```python
from build123d import *

# Parameters (mm, degrees)
SKETCH_1_W             = 23.5
SKETCH_1_H             = 12
EXTRUDE_1_DEPTH        = 771
HOLE_WIZARD_M6_1_D     = 5
HOLE_WIZARD_M6_1_DEPTH = 15
HOLE_WIZARD_M6_1_TIP   = 1.502151548
HOLE_WIZARD_M6_2_D     = 5
HOLE_WIZARD_M6_2_DEPTH = 15
HOLE_WIZARD_M6_2_TIP   = 1.502151548
SKETCH_7_R             = 4.5
CUT_EXTRUDE_1_DEPTH    = 772.729227126
SKETCH_8_R             = 5
CUT_EXTRUDE_2_DEPTH    = 15
SKETCH_9_R             = 3.5
CUT_EXTRUDE_3_DEPTH    = 15
HOLE_WIZARD_M6_3_D     = 5
HOLE_WIZARD_M6_3_DEPTH = 15
HOLE_WIZARD_M6_3_TIP   = 1.502151548
HOLE_WIZARD_M6_4_D     = 5
HOLE_WIZARD_M6_4_DEPTH = 15
HOLE_WIZARD_M6_4_TIP   = 1.502151548
SKETCH_14_R            = 4.5
CUT_EXTRUDE_4_DEPTH    = 772.729227126


with BuildPart() as part:
    # 草图1 → 凸台-拉伸1 (new, symmetric)
    with BuildSketch(Plane(origin=(0, 0, 0), x_dir=(0, 0, -1), z_dir=(1, 0, 0))):
        with BuildLine():
            Line((-14, 15), (-11.5, 15))
            Line((-11.5, 15), (-11.5, 13.5))
            Line((-11.5, 13.5), (-11.4, 13.5))
            ThreePointArc((-11.4, 13.5), (-11.117157288, 13.382842712), (-11, 13.1))
            Line((-11, 13.1), (-11, 12))
            Line((-11, 12), (-9.5, 12))
            Line((-9.5, 12), (-9.5, 15))
            Line((-9.5, 15), (-8, 15))
            Line((-8, 15), (-8, 12.5))
            Line((-8, 12.5), (-5, 12.5))
            Line((-5, 12.5), (-5, 15))
            Line((-5, 15), (5, 15))
            Line((5, 15), (5, 12.5))
            Line((5, 12.5), (8, 12.5))
            Line((8, 12.5), (8, 15))
            Line((8, 15), (9.5, 15))
            Line((9.5, 15), (9.5, 12))
            Line((9.5, 12), (11, 12))
            Line((11, 12), (11, 13.1))
            ThreePointArc((11, 13.1), (11.117157288, 13.382842712), (11.4, 13.5))
            Line((11.4, 13.5), (11.5, 13.5))
            Line((11.5, 13.5), (11.5, 15))
            Line((11.5, 15), (14, 15))
            ThreePointArc((14, 15), (14.707106781, 14.707106781), (15, 14))
            Line((15, 14), (15, 8))
            Line((15, 8), (12.5, 8))
            Line((12.5, 8), (12.5, 5))
            Line((12.5, 5), (15, 5))
            Line((15, 5), (15, -5))
            Line((15, -5), (12.5, -5))
            Line((12.5, -5), (12.5, -8))
            Line((12.5, -8), (15, -8))
            Line((15, -8), (15, -14))
            ThreePointArc((15, -14), (14.707106781, -14.707106781), (14, -15))
            Line((14, -15), (11.5, -15))
            Line((11.5, -15), (11.5, -13.5))
            Line((11.5, -13.5), (11.4, -13.5))
            ThreePointArc((11.4, -13.5), (11.117157288, -13.382842712), (11, -13.1))
            Line((11, -13.1), (11, -12))
            Line((11, -12), (9.5, -12))
            Line((9.5, -12), (9.5, -15))
            Line((9.5, -15), (8, -15))
            Line((8, -15), (8, -12.5))
            Line((8, -12.5), (5, -12.5))
            Line((5, -12.5), (5, -15))
            Line((5, -15), (-5, -15))
            Line((-5, -15), (-5, -12.5))
            Line((-5, -12.5), (-8, -12.5))
            Line((-8, -12.5), (-8, -15))
            Line((-8, -15), (-9.5, -15))
            Line((-9.5, -15), (-9.5, -12))
            Line((-9.5, -12), (-11, -12))
            Line((-11, -12), (-11, -13.1))
            ThreePointArc((-11, -13.1), (-11.117157288, -13.382842712), (-11.4, -13.5))
            Line((-11.4, -13.5), (-11.5, -13.5))
            Line((-11.5, -13.5), (-11.5, -15))
            Line((-11.5, -15), (-14, -15))
            ThreePointArc((-14, -15), (-14.707106781, -14.707106781), (-15, -14))
            Line((-15, -14), (-15, 14))
            ThreePointArc((-15, 14), (-14.707106781, 14.707106781), (-14, 15))
        make_face()
        with BuildLine():
            Line((12, -10.5), (12, -8.5))
            ThreePointArc((12, -8.5), (11.853553391, -8.146446609), (11.5, -8))
            Line((11.5, -8), (-11.5, -8))
            ThreePointArc((-11.5, -8), (-11.853553391, -8.146446609), (-12, -8.5))
            Line((-12, -8.5), (-12, -10.5))
            ThreePointArc((-12, -10.5), (-11.853553391, -10.853553391), (-11.5, -11))
            Line((-11.5, -11), (11.5, -11))
            ThreePointArc((11.5, -11), (11.853553391, -10.853553391), (12, -10.5))
        make_face(mode=Mode.SUBTRACT)
        with BuildLine():
            Line((-11.5, 11), (11.5, 11))
            ThreePointArc((11.5, 11), (11.853553391, 10.853553391), (12, 10.5))
            Line((12, 10.5), (12, 8.5))
            ThreePointArc((12, 8.5), (11.853553391, 8.146446609), (11.5, 8))
            Line((11.5, 8), (-11.5, 8))
            ThreePointArc((-11.5, 8), (-11.853553391, 8.146446609), (-12, 8.5))
            Line((-12, 8.5), (-12, 10.5))
            ThreePointArc((-12, 10.5), (-11.853553391, 10.853553391), (-11.5, 11))
        make_face(mode=Mode.SUBTRACT)
        Rectangle(SKETCH_1_W, SKETCH_1_H, mode=Mode.SUBTRACT)
    extrude(amount=EXTRUDE_1_DEPTH, both=True)

    # M6 螺纹孔1
    with Locations(Plane(origin=(0, 0, -15), x_dir=(-1, 0, 0), z_dir=(0, 0, -1))):
        with Locations((751, 0), (736, 0), (-736, 0), (-751, 0)):
            Hole(HOLE_WIZARD_M6_1_D / 2, depth=HOLE_WIZARD_M6_1_DEPTH)
            with Locations((0, 0, -(HOLE_WIZARD_M6_1_DEPTH + HOLE_WIZARD_M6_1_TIP / 2))):  # 118° drill point
                Cone(0, HOLE_WIZARD_M6_1_D / 2, HOLE_WIZARD_M6_1_TIP, mode=Mode.SUBTRACT)

    # M6 螺纹孔2
    with Locations(Plane(origin=(0, 15, 0), x_dir=(-1, 0, 0), z_dir=(0, 1, 0))):
        with Locations((-751, 0), (-736, 0), (736, 0), (751, 0)):
            Hole(HOLE_WIZARD_M6_2_D / 2, depth=HOLE_WIZARD_M6_2_DEPTH)
            with Locations((0, 0, -(HOLE_WIZARD_M6_2_DEPTH + HOLE_WIZARD_M6_2_TIP / 2))):  # 118° drill point
                Cone(0, HOLE_WIZARD_M6_2_D / 2, HOLE_WIZARD_M6_2_TIP, mode=Mode.SUBTRACT)

    # 草图7 → 切除-拉伸1 (cut, through all)
    with BuildSketch(Plane.XY.offset(15)):
        with Locations((-651, 0)):
            Circle(SKETCH_7_R)
        with Locations((-221, 0)):
            Circle(SKETCH_7_R)
        with Locations((651, 0)):
            Circle(SKETCH_7_R)
        with Locations((221, 0)):
            Circle(SKETCH_7_R)
    extrude(amount=-CUT_EXTRUDE_1_DEPTH, mode=Mode.SUBTRACT)

    # 草图8 → 切除-拉伸2 (cut)
    with BuildSketch(Plane.XY.offset(15)):
        Circle(SKETCH_8_R)
        with Locations((-25, 0)):
            Circle(SKETCH_8_R)
        with Locations((25, 0)):
            Circle(SKETCH_8_R)
    extrude(amount=-CUT_EXTRUDE_2_DEPTH, mode=Mode.SUBTRACT)

    # 草图9 → 切除-拉伸3 (cut)
    with BuildSketch(Plane(origin=(0, 0, -15), x_dir=(-1, 0, 0), z_dir=(0, 0, -1))):
        Circle(SKETCH_9_R)
        with BuildLine():
            Line((27, 2.5), (27, -2.5))
            ThreePointArc((27, -2.5), (25, -4.5), (23, -2.5))
            Line((23, -2.5), (23, 2.5))
            ThreePointArc((23, 2.5), (25, 4.5), (27, 2.5))
        make_face()
        with BuildLine():
            Line((-27, 2.5), (-27, -2.5))
            ThreePointArc((-27, -2.5), (-25, -4.5), (-23, -2.5))
            Line((-23, -2.5), (-23, 2.5))
            ThreePointArc((-23, 2.5), (-25, 4.5), (-27, 2.5))
        make_face()
    extrude(amount=-CUT_EXTRUDE_3_DEPTH, mode=Mode.SUBTRACT)

    # M6 螺纹孔3
    with Locations(Plane(origin=(0, 0, -15), x_dir=(-1, 0, 0), z_dir=(0, 0, -1))):
        with Locations((411, 0), (351, 0), (321, 0), (261, 0), (-261, 0), (-321, 0), (-351, 0), (-411, 0)):
            Hole(HOLE_WIZARD_M6_3_D / 2, depth=HOLE_WIZARD_M6_3_DEPTH)
            with Locations((0, 0, -(HOLE_WIZARD_M6_3_DEPTH + HOLE_WIZARD_M6_3_TIP / 2))):  # 118° drill point
                Cone(0, HOLE_WIZARD_M6_3_D / 2, HOLE_WIZARD_M6_3_TIP, mode=Mode.SUBTRACT)

    # M6 螺纹孔4
    with Locations(Plane(origin=(0, 0, -15), x_dir=(-1, 0, 0), z_dir=(0, 0, -1))):
        with Locations((691, 0), (-691, 0)):
            Hole(HOLE_WIZARD_M6_4_D / 2, depth=HOLE_WIZARD_M6_4_DEPTH)
            with Locations((0, 0, -(HOLE_WIZARD_M6_4_DEPTH + HOLE_WIZARD_M6_4_TIP / 2))):  # 118° drill point
                Cone(0, HOLE_WIZARD_M6_4_D / 2, HOLE_WIZARD_M6_4_TIP, mode=Mode.SUBTRACT)

    # 草图14 → 切除-拉伸4 (cut, through all)
    with BuildSketch(Plane(origin=(0, 0, -15), x_dir=(-1, 0, 0), z_dir=(0, 0, -1))):
        with Locations((691, 0)):
            Circle(SKETCH_14_R)
        with Locations((-691, 0)):
            Circle(SKETCH_14_R)
    extrude(amount=-CUT_EXTRUDE_4_DEPTH, mode=Mode.SUBTRACT)


solid = part.part
```
Check sheet for the modelled part. Datum: model origin and axes. Units: mm. A direction names the side the tool comes from. Give positions to 0.01 mm unless a question says otherwise; leave off trailing zeros. Use CSV: the item, a comma, the result in double quotes. Start each with the question number.
1) Set-up check for faces 3 (the face through (771, 7, 0)), 4 (the face through (11, -6, 0)): record each of +Z, -Z, +X, -X, +Y, -Y from which the full face is reachable in a straight line by a thin tool's end or side.
2) Material ranges on line 1 (Y direction, x = -178.5, z = -4); line 2 (Y direction, x = 201.5, z = -5.5); line 3 (Z direction, x = 39, y = 13.75), recorded low to high. Write a range as from..to.
3) Go/stop test with flat-tipped pins: P1, Ø1.5, axis at x = -476, z = 6.5, coming from the +Y side; P2, Ø5.5, axis at x = -691, y = 0, coming from the +Z side. Record where each tip stops, or that it passes through.
4) Sectioned sample at A-A, the plane x = -121. Give the number of separate pieces and of enclosed holes in the cut face, plus the area to 3 significant figures.
5) Mould release check, pull along Y, two halves, no side actions. Record for faces 1 (the face through (-771, 7, 0)), 2 (the face through (11, 6, 0)): released by +Y, released by -Y, zero draft, split by the parting line, or undercut.
Recorded:
1,face 3,"+Z, -Z, +X, +Y, -Y"
1,face 4,"+X, -X"
2,line 1,"-15..-11, -8..-6, 6..8, 11..15"
2,line 2,"-12.5..-11, -8..-6, 6..8, 11..12.5"
2,line 3,"-15..-11.5, -9.5..-8, -5..5, 8..9.5, 11.5..15"
3,P1,"y = 12.5"
3,P2,"through"
4,separate pieces,"1"
4,enclosed holes,"3"
4,area,"407 mm2"
5,face 1,"zero draft"
5,face 2,"undercut"
